Here's the drawing with two shaded views (mm, measured from the low corner). I have some questions. A direction names the side the tool comes from. Coordinates: 2 decimals unless noted, no trailing zeros. Write each loop counter-clockwise with the first axis right and the second up, starting at its lowest first coordinate (ties: lowest second). Pieces come first, ordered by that corner, then holes. Notation, with made-up numbers: (29.5, -28) - (43.5, -28) arc R14 cw to (43.5, -10) - close; hole circle Ø3 at (29.25, 72). An arc over 180 degrees is marked (long way). Answer in a Markdown table with one row per item. Add a question column.
Item 1: Which directions (+Z, -Z, +X, -X, +Y, -Y) give clear straight access to the entire face, cutting with the end or side of a thin tool? Please do the marked faces 1 and 2.
Item 2: Imagine slicing it at C-C (x = 8). Please give me the cut outline in (y, z), plus the area to 3 significant figures.
Item 3: Imagine slicing it at B-B (z = 2). Please give me the cut outline in (x, y), plus the area to 3 significant figures.
Item 4: If I drill on probe 1 along Y at (x, z) = (5, 7.25); probe 2 along Y at (x, z) = (6, 3.75); probe 3 along X at (y, z) = (7.5, 19), over which ranges is the centre line in solid material (lowest first)? Write a range as from..to.
Item 5: I'm going to push flat-ended pins straight in: pin 1 (5 mm diameter, centred on x = 17.5, z = 16.5, fed in from -Y); pin 2 (4 mm diameter, centred on x = 4.5, y = 10, fed in from +Z); pin 3 (5 mm diameter, centred on x = 13, z = 10.5, fed in from +Y). Where does each tip first touch, or does it pass through?
Item 6: We'd pull the mould along Y, two halves only. Please class the marked faces 3, 4, 5 and 6: +Y half, -Y half, draft (parallel to the pull), parting line (faces both ways), or undercut.
Item 7: Imagine slicing it at A-A (x = 5). Please give me the cut outline in (y, z), plus the area to 3 significant figures.
Item 8: Imagine slicing it at D-D (y = 1.5). Please give me the cut outline in (x, z).
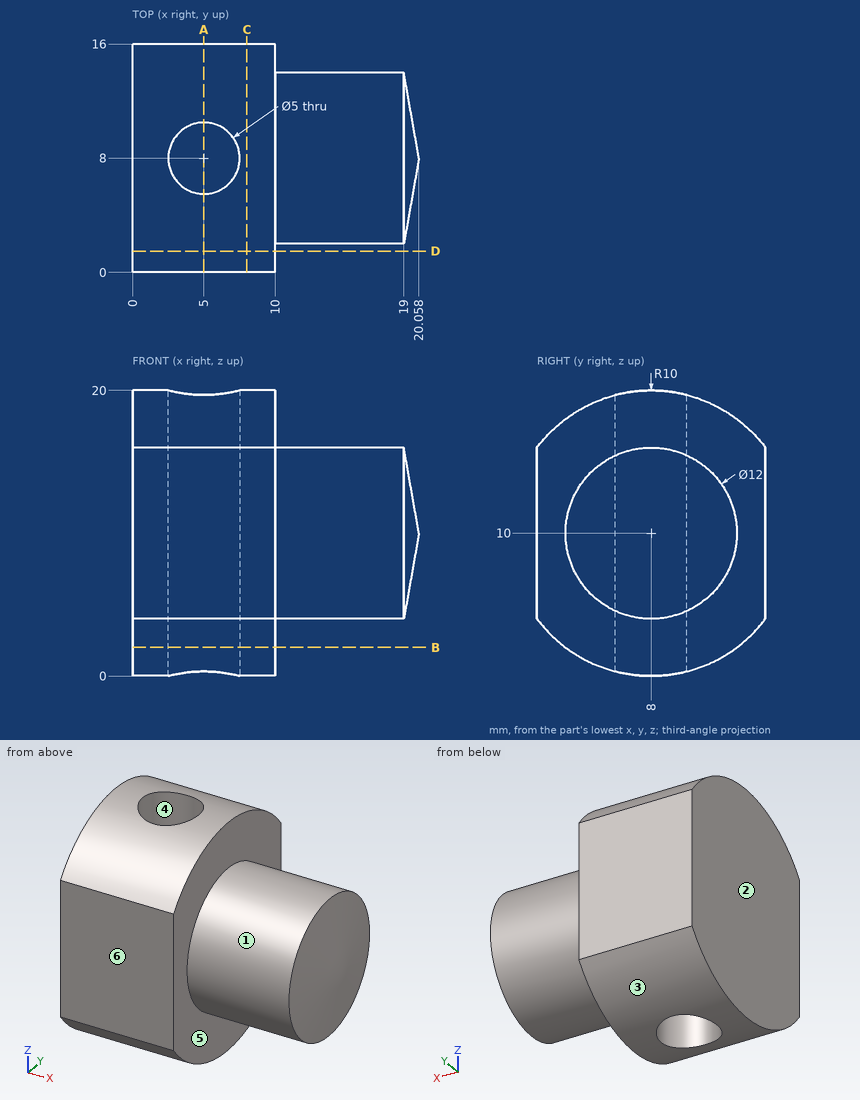
Here are the results:
| question | item | result |
|---|---|---|
| 1 | face 1 | +X |
| 1 | face 2 | +Z, -Z, -X, +Y, -Y |
| 2 | outline | (0, 4) arc R10 ccw to (16, 4) - (16, 16) arc R10 ccw to (0, 16) - close |
| 2 | area | 281 mm2 |
| 3 | outline | (0, 2) - (10, 2) - (10, 14) - (0, 14) - close; hole circle Ø5 at (5, 8) |
| 3 | area | 100 mm2 |
| 4 | probe 1 | y = 0..5.5, 10.5..16 |
| 4 | probe 2 | y = 0.19..5.71, 10.29..15.81 |
| 4 | probe 3 | x = 0..2.55, 7.45..10 |
| 5 | pin 1 | stops at y = 3.53 |
| 5 | pin 2 | stops at z = 19.94 |
| 5 | pin 3 | stops at y = 14 |
| 6 | face 3 | parting line |
| 6 | face 4 | undercut |
| 6 | face 5 | draft |
| 6 | face 6 | -Y half |
| 7 | outline | (0, 4) arc R10 ccw to (5.5, 0.32) - (5.5, 19.68) arc R10 ccw to (0, 16) - close; (10.5, 0.32) arc R10 ccw to (16, 4) - (16, 16) arc R10 ccw to (10.5, 19.68) - close |
| 7 | area | 183 mm2 |
| 8 | outline | (0, 2.4) - (10, 2.4) - (10, 17.6) - (0, 17.6) - close |
